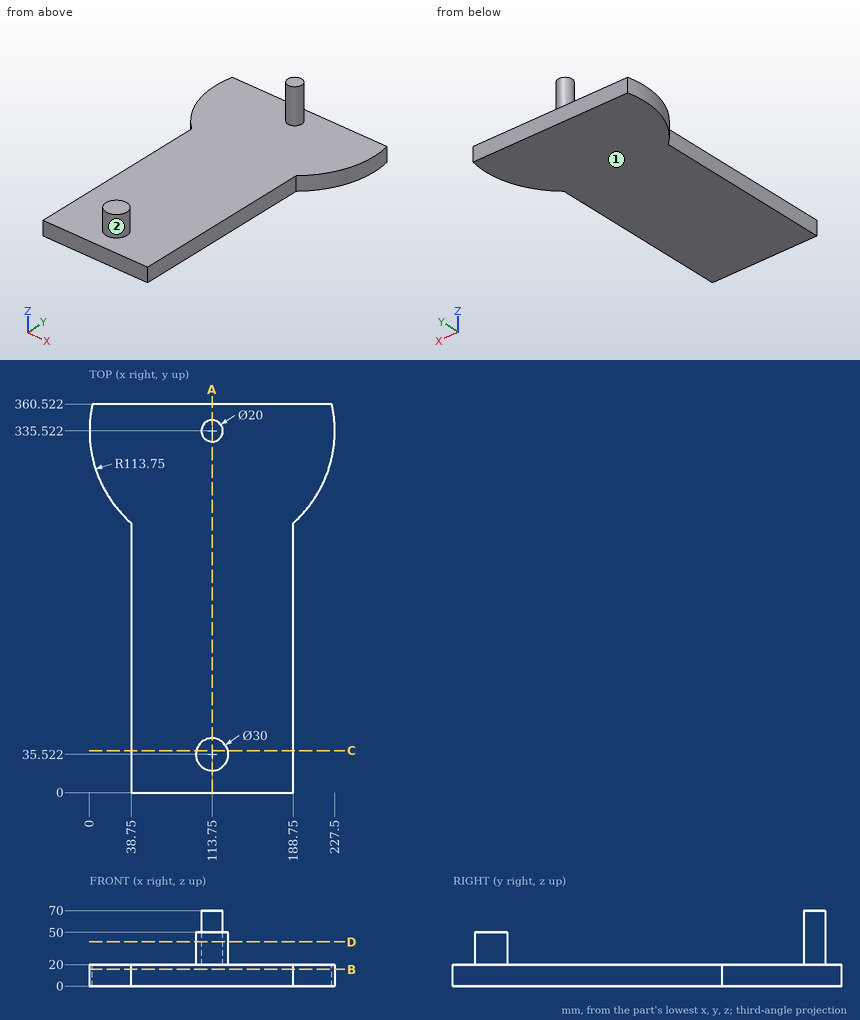
Answer from the drawing. Dimensions are ordinates in mm from the lowest x, y and z of the part. Give positions to 0.01 mm unless a question says otherwise; leave off trailing zeros. Order: outer loops, then holes, each group sorted by start corner. A loop starts at its lowest first (then second) coordinate and runs counter-clockwise, first axis right, second up. Notation, with made-up numbers: (-11, 88) - (-2, 88) arc R28 ccw to (-2, 125) - close; hole circle Ø5 at (49, 7). An arc over 180 degrees is marked (long way). One line per item, written item: value. Start each with the question number.
1. For a pull along Y with two mould halves and no side action, classify the marked faces 1 and 2 as released by +Y, released by -Y, zero draft, split by the parting line, or undercut.
2. Section D-D, the plane z = 41 is taken. Write down the section's boundary in (x, y), then the cut area to 3 significant figures.
3. Section C-C, the plane y = 39 is taken. Write down the section's boundary in (x, z).
4. Consider line 1 (Z direction, x = 54, y = 114); line 2 (X direction, y = 337, z = 16.5); line 3 (X direction, y = 215, z = 5). Determine where each line is inside the solid, lowest interval first.
5. Section A-A, the plane x = 113.75 is taken. Write down the section's boundary in (y, z).
6. Each of these flat-tipped pins is pushed along its axis until it touches: pin 1 Ø5 at (y, z) = (42, 50) entering from +X; pin 2 Ø15 at (x, y) = (112.5, 36.5) entering from +Z; pin 3 Ø16 at (y, z) = (165, 9) entering from -X. Where does it stop, or does it pass through?
7. Section B-B, the plane z = 15.5 is taken. Write down the section's boundary in (x, y).
Filled sheet:
1. face 1: zero draft
1. face 2: undercut
2. outline: circle Ø30 at (113.75, 35.52); circle Ø20 at (113.75, 335.52)
2. area: 1,020 mm²
3. outline: (38.75, 0) - (188.75, 0) - (188.75, 20) - (128.34, 20) - (128.34, 50) - (99.16, 50) - (99.16, 20) - (38.75, 20) - close
4. line 1: 0 to 20
4. line 2: 0.01 to 227.49
4. line 3: 38.75 to 188.75
5. outline: (0, 0) - (360.52, 0) - (360.52, 20) - (345.52, 20) - (345.52, 70) - (325.52, 70) - (325.52, 20) - (50.52, 20) - (50.52, 50) - (20.52, 50) - (20.52, 20) - (0, 20) - close
6. pin 1: x = 128.21
6. pin 2: z = 50
6. pin 3: x = 38.75
7. outline: (2.78, 360.52) arc R113.75 ccw to (38.75, 250) - (38.75, 0) - (188.75, 0) - (188.75, 250) arc R113.75 ccw to (224.72, 360.52) - close
